Part model, mm, in its own coordinate system. A direction names the side the tool comes from. Round coordinates to 2 decimals unless told otherwise and drop trailing zeros. Loops run counter-clockwise (first coordinate to the right, second up) from the corner with the lowest first, then second, coordinate; pieces in that order, holes last. Notation, with made-up numbers: (78.25, 58.25) -> (99.25, 58.25) arc R13 cw to (99.25, 69.25) -> close; hole circle Ø10 at (22.25, 69.5). An arc over 180 degrees is marked (long way). Answer as CSV lines item,"result".
from build123d import *

# Parameters (mm, degrees)
SKETCH1_W           = 20
SKETCH1_H           = 12
BOSS_EXTRUDE1_DEPTH = 6
SKETCH2_W           = 6
SKETCH2_H           = 18
CUT_EXTRUDE1_DEPTH  = 10


with BuildPart() as part:
    # Sketch1 → Boss-Extrude1 (new body)
    with BuildSketch(Plane.XY):
        with BuildLine():
            Line((211.428617248, -24.317756725), (162.653205504, 19.127417073))
            ThreePointArc((162.653205504, 19.127417073), (74.134115414, 34.8851986), (24.686380191, -40.207134366))
            Line((24.686380191, -40.207134366), (24.686380191, -59.317756725))
            Line((24.686380191, -59.317756725), (39.581295698, -59.317756725))
            Line((39.581295698, -59.317756725), (39.581295698, -40.207134366))
            ThreePointArc((39.581295698, -40.207134366), (116.085216489, 25.939025685), (170.486001767, -59.317756725))
            Line((170.486001767, -59.317756725), (211.428617248, -59.317756725))
            Line((211.428617248, -59.317756725), (211.428617248, -24.317756725))
        make_face()
        with Locations((192.683627049, -38.317756725)):
            Rectangle(SKETCH1_W, SKETCH1_H, mode=Mode.SUBTRACT)
    extrude(amount=BOSS_EXTRUDE1_DEPTH)

    # Sketch2 → Cut-Extrude1 (cut)
    with BuildSketch(Plane(origin=(0, 0, 0), x_dir=(-1, 0, 0), z_dir=(0, 0, -1))):
        with Locations((-32.133837945, -44.317756725)):
            Rectangle(SKETCH2_W, SKETCH2_H)
    extrude(amount=-CUT_EXTRUDE1_DEPTH, mode=Mode.SUBTRACT)


solid = part.part
Q1. Which spindle directions (+Z, -Z, +X, -X, +Y, -Y) get a long thin tool onto all of the face, cutting with end or side? Do faces 4 (the face through (125, 25, 0)), 5 (the face through (182.684, -38, 3)), 6 (the face through (39.581, -50, 3)). Say none if no direction does.
Geometry results:
face 4,"-Z, +X, -X, +Y, -Y"
face 5,"+Z, -Z"
face 6,"+Z, -Z, -Y"
Q2. Saw through at A-A, the plane y = 16. Write the cut outline in (x, z).
Geometry results:
outline,"(47.08, 0) -> (70.24, 0) -> (70.24, 6) -> (47.08, 6) -> close; (142.61, 0) -> (166.16, 0) -> (166.16, 6) -> (142.61, 6) -> close"
Q3. Saw through at C-C, the plane y = -49.5. Write the cut outline in (x, z).
Geometry results:
outline,"(24.69, 0) -> (29.13, 0) -> (29.13, 6) -> (24.69, 6) -> close; (35.13, 0) -> (39.58, 0) -> (39.58, 6) -> (35.13, 6) -> close; (172.63, 0) -> (211.43, 0) -> (211.43, 6) -> (172.63, 6) -> close"
Q4. Saw through at B-B, the plane z = 1. Write the cut outline in (x, y).
Geometry results:
outline,"(24.69, -59.32) -> (39.58, -59.32) -> (39.58, -40.21) arc R66.85 cw (long way) to (170.49, -59.32) -> (211.43, -59.32) -> (211.43, -24.32) -> (162.65, 19.13) arc R81.74 ccw to (24.69, -40.21) -> close; hole (29.13, -53.32) -> (35.13, -53.32) -> (35.13, -35.32) -> (29.13, -35.32) -> close; hole (182.68, -44.32) -> (202.68, -44.32) -> (202.68, -32.32) -> (182.68, -32.32) -> close"
Q5. Two-plate mould, pull along Y, no slides. Class faces 1 (the face through (191, -59.318, 3)), 2 (the face through (211.429, -42, 3)), 3 (the face through (202.684, -38, 3)): pulls with the +Y half, pulls with the -Y half, needs draft (parallel to the pull), parting line crosses it, or undercut.
Geometry results:
face 1,"pulls with the -Y half"
face 2,"needs draft"
face 3,"undercut"
Q6. Saw through at D-D, the plane x = 192.5. Write the cut outline in (y, z).
Geometry results:
outline,"(-59.32, 0) -> (-44.32, 0) -> (-44.32, 6) -> (-59.32, 6) -> close; (-32.32, 0) -> (-7.46, 0) -> (-7.46, 6) -> (-32.32, 6) -> close"
Q7. Drill centre lines: line 1 along X through (y, z) = (-42, 5.65); line 2 along X through (y, z) = (-40.5, 3.25); line 3 along Y through (x, z) = (106.5, 5.55). Where is each one in solid material? Low to high.
Geometry results:
line 1,"24.69 to 29.13, 35.13 to 39.58, 173.25 to 182.68, 202.68 to 211.43"
line 2,"24.69 to 29.13, 35.13 to 39.58, 173.28 to 182.68, 202.68 to 211.43"
line 3,"26.64 to 41.54"
Q8. Drop flat-ended pins along their axis: P1, Ø1.8, axis at x = 31.5, z = 2, coming from the +Y side; P2, Ø1, axis at y = -16, z = 4.5, coming from the -X side; P3, Ø3, axis at x = 190, z = 1.5, coming from the +Y side. Give the stop position or say it passes through.
Geometry results:
P1,"y = -5.54"
P2,"x = 28.2"
P3,"y = -3.89"
